Source: CAD feature listing. Evaluate the final solid. Frame: model axes, mm. Face numbers are marked on the shaded views. A direction names the side the tool comes from. Give positions to 0.01 mm unless a question says otherwise; leave off trailing zeros. Order: outer loops, then holes, each group sorted by start corner. A loop starts at its lowest first (then second) coordinate and runs counter-clockwise, first axis right, second up. Notation, with made-up numbers: M 43.25,19.5 L 99.25,19.5 A35 ccw 99.25,57.5 Z; hole C 64.5,-36 d7. An arc over 180 degrees is marked long. One line per question, with ' | ' between items. Start each with the question number.
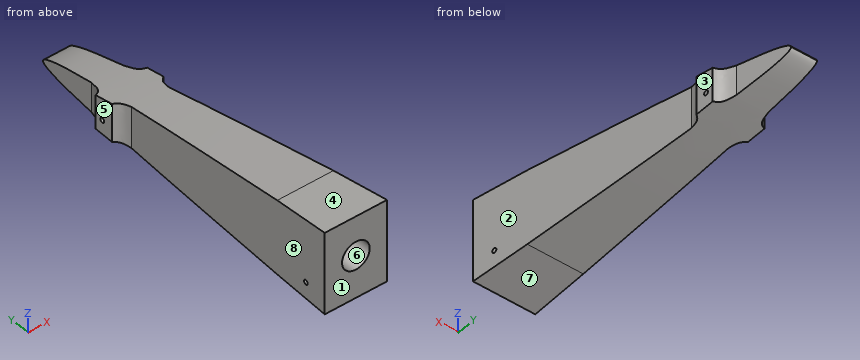
from build123d import *

# Parameters (mm, degrees)
F1_DEPTH = 21.43125
F2_R     = 9.525
F3_DEPTH = 50.8
F4_R     = 1.5875
F6_DEPTH = 42.8635
F7_DEPTH = 61.7368760046


with BuildPart() as f1:
    # F0 (on Right) → F1 (new body, symmetric)
    with BuildSketch(Plane.YZ):
        Polygon((-152.4, 69.85), (-152.4, 0), (152.4, 0), (152.4, 19.05), align=None)
    extrude(amount=F1_DEPTH, both=True)

    # F2 (on face) → F3 (cut)
    with BuildSketch(Plane.XZ.offset(152.4)):
        with Locations((0, 34.925)):
            Circle(F2_R)
    extrude(amount=-F3_DEPTH, mode=Mode.SUBTRACT)

    # F4 (on face) → F6 (intersect, through all)
    with BuildSketch(Plane.YZ.offset(21.43125)):
        with BuildLine():
            add(Edge.make_bspline(
                [(-110.784560442, 56.6772185266), (-7.8078894531, 41.1616744021), (197.1659329213, 10.2781708389), (-8.1241632402, 7.4820430193), (-110.2786958218, 6.0906601138)],
                knots=[0, 0, 0, 0, 0.5023893773, 1, 1, 1, 1], degree=3))
            Line((-110.784560442, 56.6772185266), (-152.4, 61.7358759046))
            Line((-152.4, 61.7358759046), (-152.4, 6.0906601138))
            Line((-152.4, 6.0906601138), (-135.8959368267, 6.0906601138))
            Line((-135.8959368267, 6.0906601138), (-110.2786958218, 6.0906601138))
        make_face()
        with BuildLine():
            ThreePointArc((-134.2849996434, 17.202987096), (-134.7582847356, 16.0721991454), (-135.8959368267, 15.6156601138))
            ThreePointArc((-135.8959368267, 15.6156601138), (-136.9867145512, 18.3337750467), (-134.2849996434, 17.202987096))
        make_face(mode=Mode.SUBTRACT)
        with Locations((35.1882949471, 18.7812717256)):
            Circle(F4_R, mode=Mode.SUBTRACT)
    extrude(amount=-F6_DEPTH, mode=Mode.INTERSECT)

    # F5 (on face) → F7 (intersect, through all)
    with BuildSketch(Plane(origin=(0, 0, 0), x_dir=(1, 0, 0), z_dir=(0, 0, -1))):
        with BuildLine():
            Line((21.43125, 152.4), (-21.43125, 152.4))
            Line((-21.43125, 152.4), (-12.8599264801, -17.1176383792))
            add(Edge.make_bspline(
                [(-17.78, -27.2766537964), (-16.5623446124, -26.2978531998), (-13.865051172, -24.1296597555), (-13.2159822939, -19.6015799215), (-12.8599264801, -17.1176383792)],
                knots=[0, 0, 0, 0, 0.4514360097, 1, 1, 1, 1], degree=3))
            Line((-17.78, -27.2766537964), (-17.78, -40.6726039946))
            add(Edge.make_bspline(
                [(-17.78, -40.6726039946), (-16.3984452114, -41.2366877132), (-13.0146417293, -42.6182821799), (-11.8044986652, -48.6084287427), (-11.0884383555, -52.1528908229)],
                knots=[0, 0, 0, 0, 0.4082845815, 1, 1, 1, 1], degree=3))
            Line((-11.0884383555, -52.1528908229), (-8.9427102357, -94.5896))
            Line((-8.9427102357, -94.5896), (8.9427102357, -94.5896))
            Line((8.9427102357, -94.5896), (11.0884383555, -52.1528908229))
            add(Edge.make_bspline(
                [(17.78, -40.6726039946), (16.3984452114, -41.2366877132), (13.0146417293, -42.6182821799), (11.8044986652, -48.6084287427), (11.0884383555, -52.1528908229)],
                knots=[0, 0, 0, 0, 0.4082845815, 1, 1, 1, 1], degree=3))
            Line((17.78, -40.6726039946), (17.78, -27.2766537964))
            add(Edge.make_bspline(
                [(17.78, -27.2766537964), (16.5623446124, -26.2978531998), (13.865051172, -24.1296597555), (13.2159822939, -19.6015799215), (12.8599264801, -17.1176383792)],
                knots=[0, 0, 0, 0, 0.4514360097, 1, 1, 1, 1], degree=3))
            Line((12.8599264801, -17.1176383792), (21.43125, 152.4))
        make_face()
    extrude(amount=-F7_DEPTH, mode=Mode.INTERSECT)


solid = f1.part
Item 1: Reachability of the marked faces 1, 2, 3, 4 and 5 from +Z, -Z, +X, -X, +Y, -Y: full face, straight path, thin tool, end or side. Return the list, or none.
Item 2: Pin query (flat end, axial travel): pin 1 Ø4 at (y, z) = (34, 20.5) entering from -X; pin 2 Ø8 at (y, z) = (-121.5, 39) entering from +X; pin 3 Ø4 at (y, z) = (-135.87, 17.2) entering from -X. Return the tip coordinate at first contact, or that it passes through.
Item 3: Cut plane B-B on x = 0. Count the separate pieces of the cut face and the enclosed holes in it, and give its area (3 significant figures).
Item 4: Line query: line 1 (Y direction, x = 2, z = 18); line 2 (X direction, y = 38, z = 32); line 3 (X direction, y = -118.5, z = 29). Output: solid intervals per line, ascending.
Item 5: Cut plane A-A on y = -125. Return the cut outline in (x, z) (3 decimals), and give its area (3 significant figures).
Item 6: Mould query, pull axis X, two halves, no side actions, for the marked faces 6, 7 and 8. Classes: pulls with the +X half, pulls with the -X half, needs draft (parallel to the pull), parting line crosses it, or undercut.
Results are:
1) face 1: +Z, -Z, +X, -X, -Y | face 2: +Z, -Z, +X | face 3: +Z, -Z, +X, +Y | face 4: +Z, +X, -X, +Y | face 5: +Z, -Z, -X, +Y
2) pin 1: stops at x = -17.78 | pin 2: stops at x = 20.07 | pin 3: stops at x = -20.7
3) separate pieces: 1 | enclosed holes: 2 | area: 7,720 mm2
4) line 1: y = -152.4 to -137.25, -134.5 to 33.81, 36.57 to 94.37 | line 2: x = -17.78 to 17.78 | line 3: x = -19.72 to -7.46, 7.46 to 19.72
5) outline: M -20.046,6.091 L 20.046,6.091 L 20.046,58.405 L -20.046,58.405 Z; hole C 0,34.925 d19.05 | area: 1,810 mm2
6) face 6: undercut | face 7: needs draft | face 8: pulls with the -X half
